Here's how the part is built. I have some questions about the finished solid (model axes, mm). Face numbers are marked on the shaded views. A direction names the side the tool comes from. Round coordinates to 2 decimals unless told otherwise and drop trailing zeros. Write each loop counter-clockwise with the first axis right and the second up, starting at its lowest first coordinate (ties: lowest second). Pieces come first, ordered by that corner, then holes. Notation, with made-up numbers: (80.25, 27) -> (120.25, 27) arc R31 cw to (120.25, 65) -> close; hole circle Ø8 at (49, 62). An arc over 180 degrees is marked (long way). Answer as CSV lines item,"result".
```python
from build123d import *

# Parameters (mm, degrees)
SKETCH_1_R          = 9
EXTRUDE_1_DEPTH     = 10
SKETCH_2_R          = 6.78
EXTRUDE_2_DEPTH     = 11
SKETCH_3_R          = 9
EXTRUDE_3_DEPTH     = 2
SKETCH_5_R          = 2.5
CUT_EXTRUDE_1_DEPTH = 27.286878856
SKETCH_6_R          = 1.5
CUT_EXTRUDE_2_DEPTH = 27.286878856
SKETCH_7_R          = 1.5
CUT_EXTRUDE_3_DEPTH = 27.286879012


with BuildPart() as part:
    # 草图1 → 凸台-拉伸1 (new body)
    with BuildSketch(Plane(origin=(0, 0, 0), x_dir=(1, 0, 0), z_dir=(0, 1, 0))):
        with Locations(Location((0, 0, 0), (0, 0, 270))):
            Circle(SKETCH_1_R)
    extrude(amount=EXTRUDE_1_DEPTH)

    # 草图2 → 凸台-拉伸2 (add)
    with BuildSketch(Plane(origin=(0, 10, 0), x_dir=(1, 0, 0), z_dir=(0, 1, 0))):
        with Locations(Location((0, 0, 0), (0, 0, 270))):
            Circle(SKETCH_2_R)
    extrude(amount=EXTRUDE_2_DEPTH)

    # 草图3 → 凸台-拉伸3 (add)
    with BuildSketch(Plane(origin=(0, 21, 0), x_dir=(1, 0, 0), z_dir=(0, 1, 0))):
        with Locations(Location((0, 0, 0), (0, 0, 270))):
            Circle(SKETCH_3_R)
    extrude(amount=EXTRUDE_3_DEPTH)

    # 草图5 → 切除-拉伸1 (cut, through all)
    with BuildSketch(Plane.XZ):
        with Locations(Location((0, 0, 0), (0, 0, 270))):
            Circle(SKETCH_5_R)
    extrude(amount=-CUT_EXTRUDE_1_DEPTH, mode=Mode.SUBTRACT)

    # 草图6 → 切除-拉伸2 (cut, through all)
    with BuildSketch(Plane.XY):
        with Locations(Location((0, 6, 0), (0, 0, 90))):
            Circle(SKETCH_6_R)
    extrude(amount=-CUT_EXTRUDE_2_DEPTH, mode=Mode.SUBTRACT)

    # 草图7 → 切除-拉伸3 (cut, through all)
    with BuildSketch(Plane(origin=(0, 0, 0), x_dir=(0, 0, -1), z_dir=(1, 0, 0))):
        with Locations((0, 6)):
            Circle(SKETCH_7_R)
    extrude(amount=-CUT_EXTRUDE_3_DEPTH, mode=Mode.SUBTRACT)


solid = part.part
```
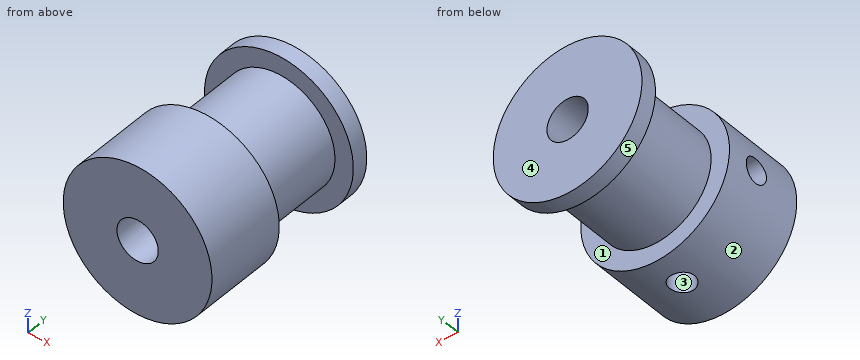
1. Suppose I cut it at D-D on z = -6. Please give me the cut outline in (x, y), and give its area (3 significant figures).
Numbers:
outline,"(-6.71, 0) -> (6.71, 0) -> (6.71, 10) -> (3.16, 10) -> (3.16, 21) -> (6.71, 21) -> (6.71, 23) -> (-6.71, 23) -> (-6.71, 21) -> (-3.16, 21) -> (-3.16, 10) -> (-6.71, 10) -> close; hole circle Ø3 at (0, 6)"
area,"223 mm^2"
2. Suppose I cut it at C-C on y = 6. Please give me the cut outline in (x, z).
Numbers:
outline,"(-8.87, -1.5) arc R9 ccw to (-1.5, -8.87) -> (-1.5, -2) arc R2.5 cw to (-2, -1.5) -> close; (-8.87, 1.5) -> (-2, 1.5) arc R2.5 cw (long way) to (1.5, -2) -> (1.5, -8.87) arc R9 ccw (long way) to start"
3. For pin 1 Ø8 at (y, z) = (10.5, 2.5) entering from -X; pin 2 Ø3 at (x, z) = (0, 0) entering from -Y; pin 3 Ø1.5 at (y, z) = (19.5, 1) entering from -X; pin 4 Ø8 at (y, z) = (16, 5.5) entering from +X, each with a flat end and sliding along its axis, tell me the tip position at first contact or that it passes through.
Numbers:
pin 1,"stops at x = -9"
pin 2,"passes through"
pin 3,"stops at x = -6.78"
pin 4,"stops at x = 6.61"
4. If I drill on line 1 (X direction, y = 15.25, z = 0); line 2 (Y direction, x = 3.25, z = 7); line 3 (Y direction, x = -6, z = 0), over which ranges is the centre line in solid material (lowest first)?
Numbers:
line 1,"x = -6.78 to -2.5, 2.5 to 6.78"
line 2,"y = 0 to 10, 21 to 23"
line 3,"y = 0 to 4.5, 7.5 to 23"
5. Suppose I cut it at B-B on z = 0. Please give me the cut outline in (x, y).
Numbers:
outline,"(-9, 0) -> (-2.5, 0) -> (-2.5, 4.5) -> (-9, 4.5) -> close; (-9, 7.5) -> (-2.5, 7.5) -> (-2.5, 23) -> (-9, 23) -> (-9, 21) -> (-6.78, 21) -> (-6.78, 10) -> (-9, 10) -> close; (2.5, 0) -> (9, 0) -> (9, 10) -> (6.78, 10) -> (6.78, 21) -> (9, 21) -> (9, 23) -> (2.5, 23) -> close"
6. If we mould it in two halves opening along Y, with no side actions, what happens to the marked faces 3, 4 and 5? For each: released by +Y, released by -Y, zero draft, split by the parting line, or undercut.
Numbers:
face 3,"undercut"
face 4,"released by +Y"
face 5,"zero draft"
7. Suppose I cut it at A-A on x = 0. Please give me the cut outline in (y, z).
Numbers:
outline,"(0, -9) -> (4.5, -9) -> (4.5, -2.5) -> (0, -2.5) -> close; (0, 2.5) -> (23, 2.5) -> (23, 9) -> (21, 9) -> (21, 6.78) -> (10, 6.78) -> (10, 9) -> (0, 9) -> close; (7.5, -9) -> (10, -9) -> (10, -6.78) -> (21, -6.78) -> (21, -9) -> (23, -9) -> (23, -2.5) -> (7.5, -2.5) -> close"
8. On a 3-axis mill with a long thin cutter (end or side, diameter ignored), from which of +Z, -Z, +X, -X, +Y, -Y can I reach the whole of each face in a straight line? I mean the marked faces 1 and 2. Say none if no direction works.
Numbers:
face 1,"none"
face 2,"+Y, -Y"
